from build123d import *

# Parameters (mm, degrees)
SKETCH1_W           = 215
SKETCH1_H           = 115
BOSS_EXTRUDE1_DEPTH = 50
SKETCH2_W           = 18
SKETCH2_H           = 112
CUT_EXTRUDE2_DEPTH  = 25
SHELL1_START        = -84.5
SHELL1_OUTLINE_W    = 45
SHELL1_OUTLINE_H    = 105
SHELL1_DEPTH        = 187
SHELL1_START_2      = -102.5
SHELL1_2_OUTLINE_W  = 20
SHELL1_2_OUTLINE_H  = 105
SHELL1_2_DEPTH      = 18


# Read off the part's stored shape, not the designer's step: Shell1
with BuildPart() as part:
    # Sketch1 → Boss-Extrude1 (new body)
    with BuildSketch(Plane(origin=(0, 0, 0), x_dir=(1, 0, 0), z_dir=(0, 1, 0))):
        Rectangle(SKETCH1_W, SKETCH1_H)
    extrude(amount=BOSS_EXTRUDE1_DEPTH)

    # Sketch2 → Cut-Extrude2 (cut)
    with BuildSketch(Plane(origin=(0, 50, 0), x_dir=(1, 0, 0), z_dir=(0, 1, 0))):
        with Locations((-98.5, 0)):
            Rectangle(SKETCH2_W, SKETCH2_H)
    extrude(amount=-CUT_EXTRUDE2_DEPTH, mode=Mode.SUBTRACT)

    # Shell1 outline → Shell1 (cut)
    with BuildSketch(Plane.YZ.offset(SHELL1_START)):
        with Locations((22.5, 0)):
            Rectangle(SHELL1_OUTLINE_W, SHELL1_OUTLINE_H)
    extrude(amount=SHELL1_DEPTH, mode=Mode.SUBTRACT)

    # Shell1 2 outline → Shell1 2 (cut)
    with BuildSketch(Plane.YZ.offset(SHELL1_START_2)):
        with Locations((10, 0)):
            Rectangle(SHELL1_2_OUTLINE_W, SHELL1_2_OUTLINE_H)
    extrude(amount=SHELL1_2_DEPTH, mode=Mode.SUBTRACT)


solid = part.part
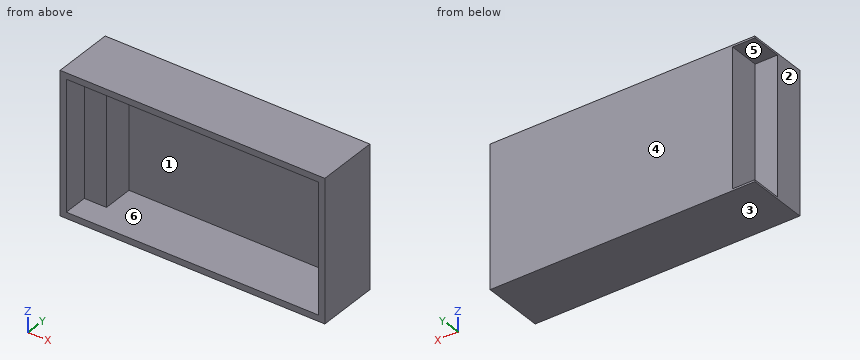
Source: CAD feature listing. Evaluate the final solid. Frame: model axes, mm. Face numbers are marked on the shaded views. A direction names the side the tool comes from. Coordinates: 2 decimals unless noted, no trailing zeros. Order: outer loops, then holes, each group sorted by start corner. A loop starts at its lowest first (then second) coordinate and runs counter-clockwise, first axis right, second up. Notation, with made-up numbers: M 1.5,-11.75 L 12.5,-11.75 A29 cw 12.5,25.25 Z; hole C 38,70.25 d6. An arc over 180 degrees is marked long. Write each question's results on one line, items separated by ' | '. Start each with the question number.
1. Section B-B, the plane x = -74. Return the cut outline in (y, z).
2. Reachability of the marked faces 4, 5 and 6 from +Z, -Z, +X, -X, +Y, -Y: full face, straight path, thin tool, end or side. Return the list, or none.
3. Section C-C, the plane y = 47.5. Return the cut outline in (x, z), then the cut area to 3 significant figures.
4. Material intervals for L1, parallel to Z at x = 21.5, y = 25; L2, parallel to X at y = 16.5, z = -36.5; L3, parallel to X at y = 40, z = -34.5, sorted ascending.
5. Draft query along Z for the marked faces 1, 2 and 3. Return one class per face: +Z half, -Z half, draft (parallel to the pull), parting line (faces both ways), or undercut.
6. Section D-D, the plane z = -36.5. Return the cut outline in (x, y), then the cut area to 4 significant figures.
7. Section A-A, the plane y = 4. Return the cut outline in (x, z).
8. Pin query (flat end, axial travel): pin 1 (4 mm diameter, centred on x = -82, z = -4.5, fed in from -Y); pin 2 (7.5 mm diameter, centred on y = 37.5, z = 22, fed in from -X); pin 3 (5.5 mm diameter, centred on x = -91.5, z = 2.5, fed in from -Y). Return the tip coordinate at first contact, or that it passes through.
Solution:
1) outline: M 0,-57.5 L 50,-57.5 L 50,57.5 L 0,57.5 L 0,52.5 L 45,52.5 L 45,-52.5 L 0,-52.5 Z
2) face 4: +Z, -Z, +X, -X, +Y | face 5: -X, +Y | face 6: -Y
3) outline: M -107.5,-57.5 L 107.5,-57.5 L 107.5,57.5 L -107.5,57.5 L -107.5,56 L -89.5,56 L -89.5,-56 L -107.5,-56 Z | area: 22,700 mm²
4) L1: -57.5 to -52.5, 52.5 to 57.5 | L2: -107.5 to -102.5, 102.5 to 107.5 | L3: -89.5 to -84.5, 102.5 to 107.5
5) face 1: undercut | face 2: draft | face 3: -Z half
6) outline: M -107.5,0 L -102.5,0 L -102.5,20 L -84.5,20 L -84.5,45 L 102.5,45 L 102.5,0 L 107.5,0 L 107.5,50 L -89.5,50 L -89.5,25 L -107.5,25 Z | area: 1,525 mm²
7) outline: M -107.5,-57.5 L 107.5,-57.5 L 107.5,57.5 L -107.5,57.5 Z; hole M -102.5,-52.5 L 102.5,-52.5 L 102.5,52.5 L -102.5,52.5 Z
8) pin 1: y = 45 | pin 2: x = -89.5 | pin 3: y = 20
